from build123d import *

# Parameters (mm, degrees)
F0_R     = 12.7
F1_DEPTH = 9.525
F2_W     = 76.2
F2_H     = 88.9
F3_DEPTH = 19.05
F4_R     = 12.7
F5_DEPTH = 19.05
F6_R     = 12.7
F7_DEPTH = 19.05


with BuildPart() as f1:
    # F0 (on Front) → F1 (new body, symmetric)
    with BuildSketch(Plane.XZ):
        with BuildLine():
            Line((-114.3, -38.1), (0, -38.1))
            ThreePointArc((0, -38.1), (38.1, 0), (0, 38.1))
            Line((0, 38.1), (-114.3, 38.1))
            ThreePointArc((-114.3, 38.1), (-143.460478, 32.29962), (-168.181537, 15.781537))
            Line((-168.181537, 15.781537), (-114.3, -38.1))
        make_face()
        Circle(F0_R, mode=Mode.SUBTRACT)
    extrude(amount=F1_DEPTH, both=True)

    # F2 (on face) → F3 (join)
    with BuildSketch(Plane(origin=(-76.2, 0, -76.2), x_dir=(0.707107, 0, -0.707107), z_dir=(-0.707107, 0, -0.707107))):
        with Locations((-91.981537, 0)):
            Rectangle(F2_W, F2_H)
    extrude(amount=F3_DEPTH)

    # F4 (on face) → F5 (join)
    with BuildSketch(Plane.XZ.offset(44.45)):
        with BuildLine():
            ThreePointArc((-213.082817, -29.119744), (-213.082817, -83.001281), (-159.201281, -83.001281))
            Line((-159.201281, -83.001281), (-114.3, -38.1))
            Line((-114.3, -38.1), (-168.181537, 15.781537))
            Line((-168.181537, 15.781537), (-213.082817, -29.119744))
        make_face()
        with Locations((-186.142049, -56.060512)):
            Circle(F4_R, mode=Mode.SUBTRACT)
    extrude(amount=-F5_DEPTH)

    # F6 (on face) → F7 (join)
    with BuildSketch(Plane(origin=(0, 44.45, 0), x_dir=(-1, 0, 0), z_dir=(0, 1, 0))):
        with BuildLine():
            Line((213.082817, -29.119744), (168.181537, 15.781537))
            Line((168.181537, 15.781537), (114.3, -38.1))
            Line((114.3, -38.1), (159.201281, -83.001281))
            ThreePointArc((159.201281, -83.001281), (213.082817, -83.001281), (213.082817, -29.119744))
        make_face()
        with Locations((186.142049, -56.060512)):
            Circle(F6_R, mode=Mode.SUBTRACT)
    extrude(amount=-F7_DEPTH)


solid = f1.part
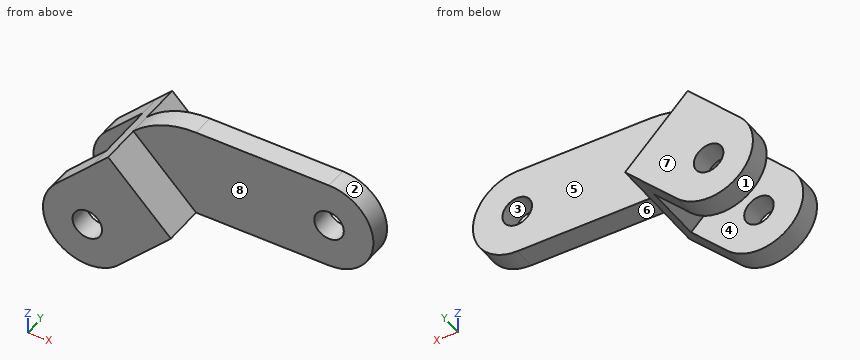
Source: CAD feature listing. Evaluate the final solid. Frame: model axes, mm. Face numbers are marked on the shaded views. A direction names the side the tool comes from. Round coordinates to 2 decimals unless told otherwise and drop trailing zeros. Order: outer loops, then holes, each group sorted by start corner. A loop starts at its lowest first (then second) coordinate and runs counter-clockwise, first axis right, second up. Notation, with made-up numbers: (-24, 87) - (6, 87) arc R21 cw to (6, 122) - close; hole circle Ø6 at (-26, 48.5). An arc over 180 degrees is marked (long way). Use a Markdown table: item, result. Add a question column.
1. Section query B-B (x = -176.5). Return the cut outline in (y, z), then the cut area to 3 significant figures.
2. First-contact query: pin 1 (23 mm diameter, centred on x = -89.5, z = -16, fed in from +Y) (3 decimals); pin 2 (8 mm diameter, centred on y = 5.5, z = -32, fed in from -X); pin 3 (12 mm diameter, centred on x = -139.5, z = 22, fed in from -Y) (3 decimals); pin 4 (15 mm diameter, centred on x = -186.14, z = -56.06, fed in from -Y). Flat tips, straight axial feed; report the tip coordinate or a pass-through.
3. Set-up query: the marked faces 4, 5, 6, 7 and 8. Return all of +Z, -Z, +X, -X, +Y, -Y with unobstructed straight access to the full face (end or side cutting, diameter ignored); none if empty.
4. Mould query, pull axis X, two halves, no side actions, for the marked faces 1, 2 and 3. Classes: +X half, -X half, draft (parallel to the pull), parting line (faces both ways), or undercut.
5. Section query C-C (y = 36). Return the cut outline in (x, z), then the cut area to 3 significant figures.
6. Line query: probe 1 along Y at (x, z) = (-160, -71); probe 2 along Y at (x, z) = (-43, -2.5) (3 decimals); probe 3 along Z at (x, y) = (-111.5, 1). Output: solid intervals per line, ascending.
Derived:
| question | item | result |
|---|---|---|
| 1 | outline | (-44.45, -92.92) - (-25.4, -92.92) - (-25.4, -64.33) - (-44.45, -64.33) - close; (-44.45, -47.79) - (-25.4, -47.79) - (-25.4, -2.84) - (25.4, -2.84) - (25.4, -47.79) - (44.45, -47.79) - (44.45, 7.46) - (-44.45, 7.46) - close; (25.4, -92.92) - (44.45, -92.92) - (44.45, -64.33) - (25.4, -64.33) - close |
| 1 | area | 3,720 mm2 |
| 2 | pin 1 | y = 9.525 |
| 2 | pin 2 | x = -151.34 |
| 2 | pin 3 | y = -9.525 |
| 2 | pin 4 | through |
| 3 | face 4 | -Z, -X |
| 3 | face 5 | +Z, +X, +Y |
| 3 | face 6 | -Z, +X, +Y, -Y |
| 3 | face 7 | +Z, -Z, +X, -X, +Y |
| 3 | face 8 | +Z, +X, -Y |
| 4 | face 1 | parting line |
| 4 | face 2 | +X half |
| 4 | face 3 | undercut |
| 5 | outline | (-213.08, -29.12) arc R38.1 ccw to (-159.2, -83) - (-114.3, -38.1) - (-168.18, 15.78) - close; hole circle Ø25.4 at (-186.14, -56.06) |
| 5 | area | 6,610 mm2 |
| 6 | probe 1 | -44.45 to -25.4, 25.4 to 44.45 |
| 6 | probe 2 | -9.525 to 9.525 |
| 6 | probe 3 | -38.1 to 38.1 |
